Geometry: final body of the model. Coordinates: model frame, mm. A direction names the side the tool comes from. Give positions to 0.01 mm unless a question says otherwise; leave off trailing zeros. One line per question, with ' | ' between items. Start each with the question number.
Item 1: Set-up query: faces 1 (the cylindrical face through (-158.327, 3.013, 37.818)), 2 (the flat face through (162.2, 6.112, 42.2)). Return all of +Z, -Z, +X, -X, +Y, -Y with unobstructed straight access to the full face (end or side cutting, diameter ignored); none if empty.
Item 2: Material intervals for line 1 along Z through (x, y) = (-160, 7.15); line 2 along X through (y, z) = (9.2, -40); line 3 along Z through (x, y) = (-160, 4.5), sorted ascending. Write a range as [from, to].
Item 3: Pin query (flat end, axial travel): P1, Ø9, axis at x = 80, z = 40, coming from the +Y side; P2, Ø3.5, axis at x = 160, z = -40, coming from the -Y side. Return the tip coordinate at first contact, or that it passes through.
Autodesk Inventor part; units mm, degrees
ref_plane "YZ Plane" through (0, 0, 0) normal (1, 0, 0) x (0, 1, 0)
ref_plane "XZ Plane" through (0, 0, 0) normal (0, 1, 0) x (-1, 0, 0)
ref_plane "XY Plane" through (0, 0, 0) normal (0, 0, 1) x (1, 0, 0)
sketch "Sketch1" plane through (0, 0, 0) normal (0, 1, 0) x (-1, 0, 0)
  line L0 (170, 50) -> (-170, 50)
  line L1 (-170, 50) -> (-170, -50)
  line L2 (-170, -50) -> (170, -50)
  line L3 (170, -50) -> (170, 50)
  line L4 (170, 50) -> (-170, -50) construction
  line L5 (-170, 50) -> (170, -50) construction
  point P0 (0, 0)
  dimension "d0" = 340
  dimension "d1" = 100
extrude "Extrusion1" add sketch "Sketch1" along normal blind 11.1125
sketch "Sketch2" plane through (0, 11.1125, 0) normal (0, 1, 0) x (1, 0, 0)
  line L0 (-170, -50) -> (170, -50)
  line L1 (170, -50) -> (170, 50)
  line L2 (170, 50) -> (-170, 50)
  line L3 (-170, 50) -> (-170, -50)
  point P0 (0, 0)
  point P1 (-160, -40)
  dimension "d4" = 10
  dimension "d5" = 10
hole "Hole1" at (-160, 11.1125, 40) direction (0, -1, 0) diameter 5.5 end through all counterbore diameter 10 counterbore depth 5
pattern_linear "Rectangular Pattern1" count 2 spacing 80 along (0, 0, -1) count 5 spacing 80 along (1, 0, 0) of "Hole1"
sketch "Sketch3" plane through (-170, 0, -50) normal (-1, 0, 0) x (0, 0, 1)
  line L0 (0, 0) -> (100, 0)
  line L1 (100, 0) -> (100, 11.1125)
  line L2 (0, 11.1125) -> (100, 11.1125)
  line L3 (0, 0) -> (0, 11.1125)
  line L4 (0, 0) -> (0, 11.1125)
  arc A0 (0, 3.175) -> (0, 6.35) centre (0, 4.7625) ccw
  point P0 (50, 0)
  dimension "d19" = 1.5875
  dimension "d20" = 6.35
extrude "oRingGroove" cut sketch "Sketch3" against normal through all contours L3 A0
mirror "Mirror1" about plane through (0, 0, 0) normal (0, 0, 1) of "oRingGroove"
equation "\"d1\" = depth"
equation "\"d2\" = facingThickness - facingGasketThickness"
equation "\"d19\" = 0.125 * facingThickness"
equation "\"d20\" = 0.5 * facingThickness"
equation "\"mppcMountThickness\" = 6.35"
equation "\"depth\" = 100"
equation "\"facingThickness\" = 12.7"
equation "\"facingGasketThickness\" = 1.5875"
properties part number "sideFace" material "Wood (Cherry)"
Result sheet:
1) face 1: +Y, -Y | face 2: +Y
2) line 1: z = [-50, -45], [-35, 35], [45, 50] | line 2: x = [-170, -165], [-155, -85], [-75, -5], [5, 75], [85, 155], [165, 170] | line 3: z = [-48.43, -42.75], [-37.25, 37.25], [42.75, 48.43]
3) P1: stops at y = 6.11 | P2: passes through
